```python
from build123d import *

# Parameters (mm, degrees)
F0_W      = 2.5
F0_H      = 24.4
F1_DEPTH  = 25
F4_R      = 1.5
F4_R_2    = 4
F5_DEPTH  = 2.5
F6_SIZE   = 5
F10_R     = 1.5
F11_DEPTH = 60
F8_W      = 25
F8_H      = 25
F12_DEPTH = 20
F13_SIZE  = 5.19999
F15_R     = 4
F16_DEPTH = 40


# Not quite as in the source:
# - a fillet or chamfer is up to 0.001 mm smaller than in the source, because OpenCascade refuses the exact size


with BuildPart() as f1:
    # F0 (on Top) → F1 (new body)
    with BuildSketch(Plane.XY):
        Polygon((-28.4, 12.2), (-25.9, 12.2), (-25.9, 12.7), (35.9, 12.7), (35.9, -12.7), (-25.9, -12.7), (-25.9, -12.2), (-28.4, -12.2), (-28.4, -22.7), (45.9, -22.7), (45.9, 22.7), (-28.4, 22.7), align=None)
        with Locations((-27.15, 0)):
            Rectangle(F0_W, F0_H)
    extrude(amount=F1_DEPTH)

    # F4 (on offset) → F5 (cut)
    with BuildSketch(Plane.YZ.offset(-28.4)):
        with Locations((-8.5, 12.5)):
            Circle(F4_R)
        with Locations((0, 12.5)):
            Circle(F4_R_2)
        with Locations((8.5, 12.5)):
            Circle(F4_R)
    extrude(amount=F5_DEPTH, mode=Mode.SUBTRACT)

    # F6
    f6_edges = [f1.edges().sort_by_distance(p)[0] for p in [
        (45.9, 22.7, 12.5),
        (-28.4, 22.7, 12.5),
        (8.75, 22.7, 0),
        (8.75, 22.7, 25),
        (-28.4, -22.7, 12.5),
        (45.9, -22.7, 12.5),
        (8.75, -22.7, 0),
        (8.75, -22.7, 25),
    ]]
    chamfer(f6_edges, length=F6_SIZE)

    # F10 (on offset) → F11 (cut)
    with BuildSketch(Plane.XZ.offset(22.7)):
        with Locations((0, 12.1945459396)):
            Circle(F10_R)
    extrude(amount=-F11_DEPTH, mode=Mode.SUBTRACT)

    # F8 (on offset) → F12 (join)
    with BuildSketch(Plane.YZ.offset(45.9)):
        with Locations((0, 12.5)):
            Rectangle(F8_W, F8_H)
    extrude(amount=F12_DEPTH)

    # F13 (size 5.2 in the source; OpenCascade refuses exactly that, so slightly less here)
    f13_edges = [f1.edges().sort_by_distance(p)[0] for p in [
        (45.9, 12.5, 12.5),
        (45.9, -12.5, 12.5),
    ]]
    chamfer(f13_edges, length=F13_SIZE)

    # F15 (on offset) → F16 (cut)
    with BuildSketch(Plane.YZ.offset(65.9)):
        with Locations((0, 12.5)):
            Circle(F15_R)
    extrude(amount=-F16_DEPTH, mode=Mode.SUBTRACT)


solid = f1.part
```
The listing builds one solid part. Answer for the finished solid, in the listing's coordinates (mm). A direction names the side the tool comes from. Give positions to 0.01 mm unless a question says otherwise; leave off trailing zeros. Order: outer loops, then holes, each group sorted by start corner. A loop starts at its lowest first (then second) coordinate and runs counter-clockwise, first axis right, second up. Notation, with made-up numbers: (-0.75, 15.5) - (57.25, 15.5) arc R21 cw to (57.25, 27.5) - close; hole circle Ø11 at (59, -33). An arc over 180 degrees is marked (long way). Answer in a Markdown table with one row per item. Add a question column.
Q1. The part is cut by section B-B (x = -18). Determine the outline of the cut face in (y, z), then the cut area to 3 significant figures.
Q2. Find the intervals of material crossed by line 1 along Y through (x, z) = (-8, 13); line 2 along Z through (x, y) = (-27.1, -8.5); line 3 along X through (y, z) = (4, 2.5), in increasing order. Write a range as [from, to].
Q3. The part is cut by section D-D (x = 0). Determine the outline of the cut face in (y, z), then the cut area to 3 significant figures.
Q4. For a pull along Z with two mould halves and no side action, classify faces 1 (the flat face through (43.4, 20.2, 12.3)), 2 (the flat face through (8.2, -20.2, 2.5)), 3 (the cylindrical face through (51.11, -0.521, 16.466)) as released by +Z, released by -Z, zero draft, split by the parting line, or undercut.
Q5. The part is cut by section A-A (y = -5). Determine the outline of the cut face in (x, z), then the cut area to 4 significant figures.
Q6. Which of the six approach directions +Z, -Z, +X, -X, +Y, -Y give full straight-line access (tool end or side, diameter ignored) to faces 4 (the flat face through (58, 12.5, 12)), 5 (the cylindrical face through (-27.17, -10, 12.57)), 6 (the flat face through (5, -12.7, 12)), 7 (the flat face through (-25.9, 20.2, 12.3)), 8 (the flat face through (39, 0, 0))?
Q7. Given P1, Ø2.5, axis at x = 0, z = 12.19, coming from the -Y side; P2, Ø7.5, axis at x = 60.5, z = 9.5, coming from the +Y side; P3, Ø4, axis at x = 53.5, z = 15.5, coming from the -Y side; P4, Ø4, axis at y = -16, z = 21.5, coming from the +X side, each flat-ended and moving along its own axis, determine where each tip first touches the part or whether it passes through.
Determined:
| question | item | result |
|---|---|---|
| 1 | outline | (-22.7, 5) - (-17.7, 0) - (-12.7, 0) - (-12.7, 25) - (-17.7, 25) - (-22.7, 20) - close; (12.7, 0) - (17.7, 0) - (22.7, 5) - (22.7, 20) - (17.7, 25) - (12.7, 25) - close |
| 1 | area | 450 mm² |
| 2 | line 1 | y = [-22.7, -12.7], [12.7, 22.7] |
| 2 | line 2 | z = [0, 11], [14, 25] |
| 2 | line 3 | x = [-28.4, -25.9], [35.9, 65.9] |
| 3 | outline | (-22.7, 5) - (-17.7, 0) - (-12.7, 0) - (-12.7, 10.69) - (-22.7, 10.69) - close; (-22.7, 13.69) - (-12.7, 13.69) - (-12.7, 25) - (-17.7, 25) - (-22.7, 20) - close; (12.7, 0) - (17.7, 0) - (22.7, 5) - (22.7, 10.69) - (12.7, 10.69) - close; (12.7, 13.69) - (22.7, 13.69) - (22.7, 20) - (17.7, 25) - (12.7, 25) - close |
| 3 | area | 390 mm² |
| 4 | face 1 | zero draft |
| 4 | face 2 | released by -Z |
| 4 | face 3 | undercut |
| 5 | outline | (-28.4, 0) - (-25.9, 0) - (-25.9, 25) - (-28.4, 25) - close; (35.9, 0) - (65.9, 0) - (65.9, 25) - (35.9, 25) - close |
| 5 | area | 812.5 mm² |
| 6 | face 4 | +Z, -Z, +X, +Y |
| 6 | face 5 | -X |
| 6 | face 6 | +Z, -Z |
| 6 | face 7 | +Z, -Z, -X, +Y |
| 6 | face 8 | -Z, +X, -X, +Y, -Y |
| 7 | P1 | passes through |
| 7 | P2 | stops at y = 12.5 |
| 7 | P3 | stops at y = -12.5 |
| 7 | P4 | stops at x = 49.6 |
